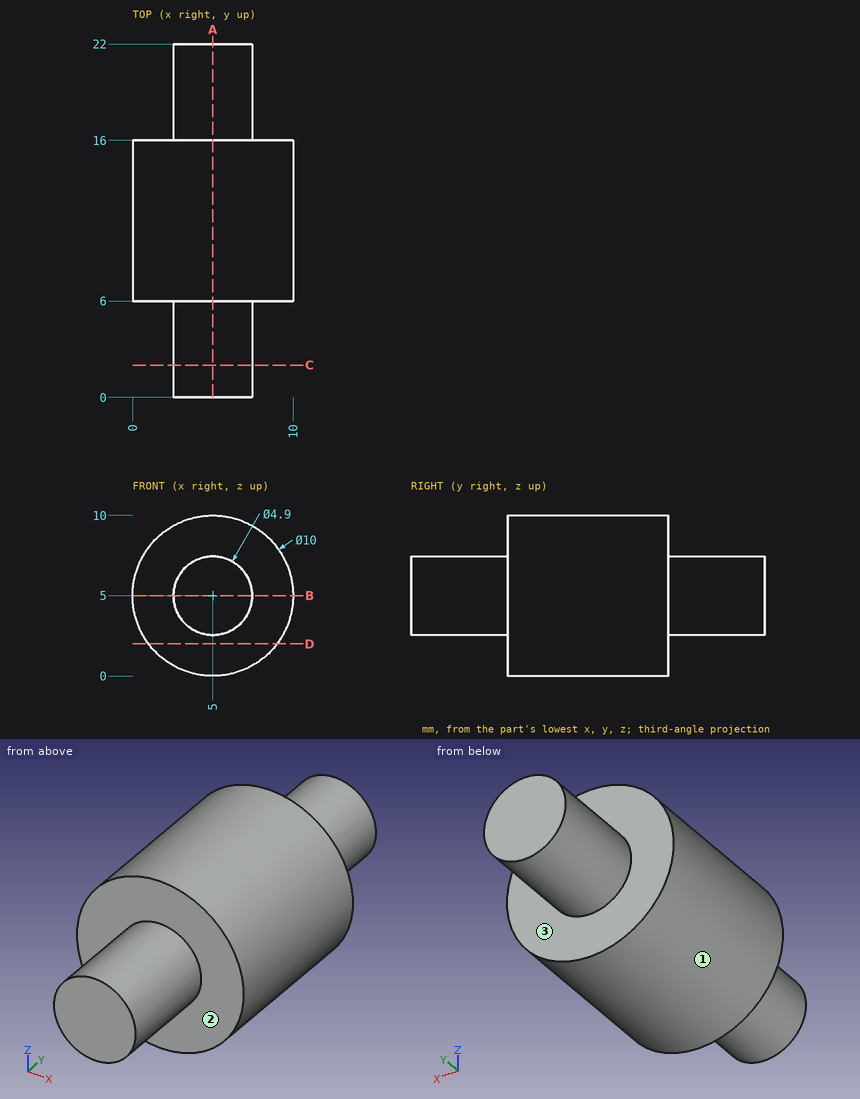
Check sheet for the drawn part. Datum: minimum x, y, z corner. Units: mm. A direction names the side the tool comes from. Give positions to 0.01 mm unless a question says otherwise; leave off trailing zeros. Write each loop counter-clockwise with the first axis right and the second up, starting at its lowest first coordinate (ties: lowest second). Pieces come first, ordered by that corner, then holes. Notation, with made-up numbers: M 73.5,-1 L 127.5,-1 A27 cw 127.5,23 Z; hole C -19,-18 d7. An arc over 180 degrees is marked long. One line per question, with ' | ' between items.
1. Cross-section at A-A (x = 5). Enter the section's corners in (y, z).
Ans:
outline: M 0,2.55 L 6,2.55 L 6,0 L 16,0 L 16,2.55 L 22,2.55 L 22,7.45 L 16,7.45 L 16,10 L 6,10 L 6,7.45 L 0,7.45 Z
2. Cross-section at B-B (z = 5). Enter the section's corners in (x, y).
Ans:
outline: M 0,6 L 2.55,6 L 2.55,0 L 7.45,0 L 7.45,6 L 10,6 L 10,16 L 7.45,16 L 7.45,22 L 2.55,22 L 2.55,16 L 0,16 Z
3. Gauge pin test, flat ends, axial feed: pin 1 (1 mm diameter, centred on x = 3.5, y = 8.5, fed in from +Z); pin 2 (4 mm diameter, centred on y = 16.5, z = 1, fed in from -X); pin 3 (3 mm diameter, centred on x = 4, z = 3.5, fed in from -Y); pin 4 (5 mm diameter, centred on x = 4.5, y = 19.5, fed in from +Z). Record the tip position at first contact, or that the pin passes through.
Ans:
pin 1: z = 9.9 | pin 2: x = 0.45 | pin 3: y = 0 | pin 4: z = 7.45
4. Set-up check for the marked faces 1, 2 and 3: record each of +Z, -Z, +X, -X, +Y, -Y from which the full face is reachable in a straight line by a thin tool's end or side.
Ans:
face 1: +Y, -Y | face 2: -Y | face 3: +Y
5. Cross-section at D-D (z = 2). Enter the section's corners in (x, y).
Ans:
outline: M 1,6 L 9,6 L 9,16 L 1,16 Z
6. Scan lines: line 1 along Y through (x, z) = (9.25, 4.75); line 2 along X through (y, z) = (15, 2.5); line 3 along X through (y, z) = (21.25, 4). Record each from-to range of solid material in increasing order. Write a range as from..to.
Ans:
line 1: 6..16 | line 2: 0.67..9.33 | line 3: 2.76..7.24
7. Cross-section at C-C (y = 2). Enter the section's corners in (x, z), plus the area to 3 significant figures.
Ans:
outline: C 5,5 d4.9 | area: 18.9 mm2
